Check sheet for the modelled part. Datum: model origin and axes. Units: mm. A direction names the side the tool comes from. Round coordinates to 2 decimals unless told otherwise and drop trailing zeros. Loops run counter-clockwise (first coordinate to the right, second up) from the corner with the lowest first, then second, coordinate; pieces in that order, holes last. Notation, with made-up numbers: (15, 31) - (33, 31) arc R29 ccw to (33, 62) - close; hole circle Ø5 at (35.5, 8.25). An arc over 180 degrees is marked (long way). Put each result on its own line as item: value. Start each with the question number.
Item 1: Section check A-A, the plane z = 6. Record the cut outline in (x, y), and give its area (3 significant figures).
Item 2: Section check D-D, the plane y = -10. Record the cut outline in (x, z).
Item 3: Tool access check on faces 5 (the cylindrical face through (8.88, -9.08, 0.71)), 6 (the flat face through (18, 0, 1)), 7 (the flat face through (0, -18, 1)). Record the directions out of +Z, -Z, +X, -X, +Y, -Y that give a thin tool (end or side, any length) a straight path to the whole face; none if there is none.
Item 4: Gauge pin test, flat ends, axial feed: pin 1 Ø3 at (x, z) = (-6.5, -24.5) entering from +Y; pin 2 Ø1 at (x, z) = (5.5, -31) entering from -Y; pin 3 Ø5.5 at (x, z) = (-11, -22.5) entering from -Y; pin 4 Ø6 at (x, y) = (0, 0) entering from -Z. Record the tip position at first contact, or that the pin passes through.
Item 5: Section check B-B, the plane z = 58. Record the cut outline in (x, y), and give its area (3 significant figures).
Item 6: Draft check along X on faces 1 (the cylindrical face through (-0.33, 2.52, -63.68)), 2 (the cylindrical face through (-4.54, -4.44, -63.32)), 3 (the cylindrical face through (-0.33, 2.52, 63.32)), 4 (the cylindrical face through (-8.88, 9.08, 0.71)). Enter one of: pulls with the +X half, pulls with the -X half, needs draft (parallel to the pull), parting line crosses it, or undercut.
Item 7: Material ranges on line 1 along Z through (x, y) = (11, -0.5); line 2 along X through (y, z) = (17.5, 17); line 3 along Y through (x, z) = (-5, -23), recorded low to high.
Item 8: Section check C-C, the plane x = 4.5. Record the cut outline in (y, z), and give its area (3 significant figures).
from build123d import *

# Parameters (mm, degrees)
F0_R     = 2.54
F1_DEPTH = 76.2
F3_R     = 12.7
F4_DEPTH = 50.8


with BuildPart() as f1:
    # F0 (on Top) → F1 (new body, symmetric)
    with BuildSketch(Plane.XY):
        with BuildLine():
            Line((0, 6.35), (0, 25.4))
            ThreePointArc((0, 25.4), (-17.960512, 17.960512), (-25.4, 0))
            Line((-25.4, 0), (-6.35, 0))
            ThreePointArc((-6.35, 0), (-4.490128, -4.490128), (0, -6.35))
            Line((0, -6.35), (0, -25.4))
            ThreePointArc((0, -25.4), (17.960512, -17.960512), (25.4, 0))
            Line((25.4, 0), (6.35, 0))
            ThreePointArc((6.35, 0), (4.490128, 4.490128), (0, 6.35))
        make_face()
        Circle(F0_R, mode=Mode.SUBTRACT)
    extrude(amount=F1_DEPTH, both=True)

    # F3 (on Top) → F4 (cut, symmetric)
    with BuildSketch(Plane.XY):
        Circle(F3_R)
    extrude(amount=F4_DEPTH, both=True, mode=Mode.SUBTRACT)


solid = f1.part
Check result:
1. outline: (-25.4, 0) - (-12.7, 0) arc R12.7 cw to (0, 12.7) - (0, 25.4) arc R25.4 ccw to start; (0, -25.4) arc R25.4 ccw to (25.4, 0) - (12.7, 0) arc R12.7 cw to (0, -12.7) - close
1. area: 760 mm²
2. outline: (0, -76.2) - (23.35, -76.2) - (23.35, 76.2) - (0, 76.2) - (0, 50.8) - (7.83, 50.8) - (7.83, -50.8) - (0, -50.8) - close
3. face 5: -X, +Y
3. face 6: +Z, -Z, +X, +Y
3. face 7: +Z, -Z, -X, -Y
4. pin 1: y = 24.9
4. pin 2: y = -24.9
4. pin 3: y = 0
4. pin 4: z = -76.2
5. outline: (-25.4, 0) - (-6.35, 0) arc R6.35 ccw to (0, -6.35) - (0, -25.4) arc R25.4 ccw to (25.4, 0) - (6.35, 0) arc R6.35 ccw to (0, 6.35) - (0, 25.4) arc R25.4 ccw to start; hole circle Ø5.08 at (0, 0)
5. area: 1,060 mm²
6. face 1: undercut
6. face 2: pulls with the -X half
6. face 3: undercut
6. face 4: pulls with the +X half
7. line 1: -76.2 to -50.8, 50.8 to 76.2
7. line 2: -18.41 to 0
7. line 3: 11.67 to 24.9
8. outline: (-25, -76.2) - (4.48, -76.2) - (4.48, -50.8) - (-11.88, -50.8) - (-11.88, 50.8) - (4.48, 50.8) - (4.48, 76.2) - (-25, 76.2) - close
8. area: 2,830 mm²
